The model under review builds one solid part; all positions refer to its coordinate system, in mm. Face numbers are marked on the shaded views. A direction names the side the tool comes from. Coordinates: 2 decimals unless noted, no trailing zeros. Loops run counter-clockwise (first coordinate to the right, second up) from the corner with the lowest first, then second, coordinate; pieces in that order, holes last. Notation, with made-up numbers: (64.5, -25) - (70.5, -25) arc R29 cw to (70.5, -2) - close; hole circle Ø6 at (32, -9). An arc over 180 degrees is marked (long way). Use a Markdown table: item, result. Add a question column.
1) To check wall thickness, follow L1, parallel to Y at x = 4.5, z = -5.5; L2, parallel to Z at x = -16, y = 23; L3, parallel to Z at x = -15.5, y = 59.5. State the ranges of each line that lie inside material, in increasing order. Write a range as [from, to].
2) For the marked faces 1 and 2, list the 3-axis set-ups (+Z, -Z, +X, -X, +Y, -Y) from which the entire face can be reached by the end or side of a thin tool; tool diameter is ignored.
3) Add section C-C, the plane x = -3. Give the boundary of the cut face in (y, z).
4) The part is to be moulded in two halves that separate along X. For the marked faces 3, 4, 5 and 6, say which applies: pulls with the +X half, pulls with the -X half, needs draft (parallel to the pull), parting line crosses it, or undercut.
5) Clearance check with flat-ended pins moving along their axes: pin 1 (1 mm diameter, centred on y = 75.5, z = -12, fed in from -X); pin 2 (7.5 mm diameter, centred on x = -5, z = 2.5, fed in from +Y). State where each tip first meets the part, or that it passes through.
6) Add section A-A, the plane x = -13.5. Give the boundary of the cut face in (y, z), and give its area (3 significant figures).
7) Add section B-B, the plane z = 6.5. Give the boundary of the cut face in (x, y).
Autodesk Inventor part; units mm, degrees
ref_plane "YZ Plane" through (0, 0, 0) normal (1, 0, 0) x (0, 1, 0)
ref_plane "XZ Plane" through (0, 0, 0) normal (0, 1, 0) x (-1, 0, 0)
ref_plane "XY Plane" through (0, 0, 0) normal (0, 0, 1) x (1, 0, 0)
sketch "Sketch1" plane through (0, 0, 0) normal (0, 1, 0) x (-1, 0, 0)
  line L0 (17.5, 15.5) -> (-17.5, 15.5)
  line L1 (-17.5, 15.5) -> (-17.5, -15.5)
  line L2 (-17.5, -15.5) -> (17.5, -15.5)
  line L3 (17.5, -15.5) -> (17.5, 15.5)
  line L4 (17.5, 15.5) -> (-17.5, -15.5) construction
  line L5 (-17.5, 15.5) -> (17.5, -15.5) construction
  line L6 (0, -15.5) -> (0, -12.5) construction
  line L7 (0, -12.5) -> (3, -12.5) construction
  circle A0 centre (3, -12.5) radius 2
  circle A1 centre (-3, -12.5) radius 2
  point P0 (0, 0)
  dimension "d0" = 35
  dimension "d1" = 31
  dimension "d5" = 3
  dimension "d6" = 3
  dimension "d7" = 4
extrude "Extrusion1" add sketch "Sketch1" along normal blind 72 contours L3 L2 L1 L0 | A0 | A1
extrude "Extrusion2" add sketch "Sketch1" along normal blind 15 from surface at 72 contours A0 | A1
fillet "Fillet1" radius 3 12 edges at (17.5, 36, 15.5) (17.5, 36, -15.5) (-17.5, 36, 15.5) (-17.5, 36, -15.5) (17.5, 72, 0) (0, 72, 15.5) (0, 72, -15.5) (-17.5, 72, 0) (17.5, 0, 0) (0, 0, 15.5) (-17.5, 0, 0) (0, 0, -15.5)
properties part number "LEMONRC 1300 - 14.8V (35C)"
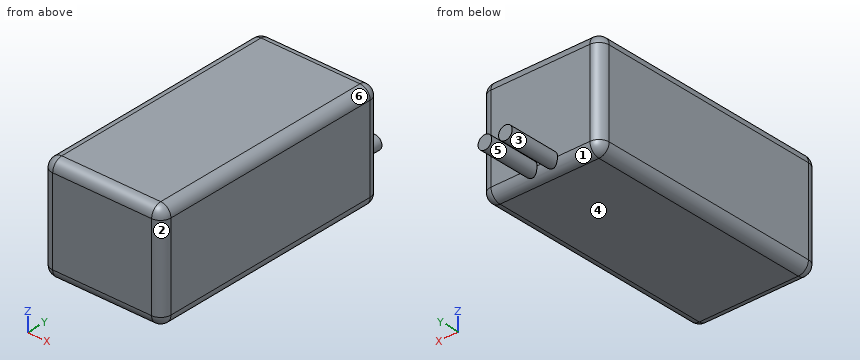
From the geometry:
| question | item | result |
|---|---|---|
| 1 | L1 | y = [0, 72] |
| 1 | L2 | z = [-15.1, 15.1] |
| 1 | L3 | z = [-15.33, 15.33] |
| 2 | face 1 | -Z, +Y |
| 2 | face 2 | +Z, -Z, +X, -Y |
| 3 | outline | (0, -12.5) arc R3 ccw to (3, -15.5) - (69, -15.5) arc R3 ccw to (71.24, -14.5) - (87, -14.5) - (87, -10.5) - (72, -10.5) - (72, 12.5) arc R3 ccw to (69, 15.5) - (3, 15.5) arc R3 ccw to (0, 12.5) - close |
| 4 | face 3 | undercut |
| 4 | face 4 | needs draft |
| 4 | face 5 | undercut |
| 4 | face 6 | pulls with the +X half |
| 5 | pin 1 | stops at x = -5 |
| 5 | pin 2 | stops at y = 72 |
| 6 | outline | (0, -12.5) arc R3 ccw to (3, -15.5) - (69, -15.5) arc R3 ccw to (72, -12.5) - (72, 12.5) arc R3 ccw to (69, 15.5) - (3, 15.5) arc R3 ccw to (0, 12.5) - close |
| 6 | area | 2,220 mm^2 |
| 7 | outline | (-17.5, 3) arc R3 ccw to (-14.5, 0) - (14.5, 0) arc R3 ccw to (17.5, 3) - (17.5, 69) arc R3 ccw to (14.5, 72) - (-14.5, 72) arc R3 ccw to (-17.5, 69) - close |
